from build123d import *

# Parameters (mm, degrees)
ESQUISSE1_R             = 2.1
BOSS_EXTRU_1_DEPTH      = 3
BOSS_EXTRU_2_START      = -50
ESQUISSE4_R             = 5
BOSS_EXTRU_2_DEPTH      = 10
ENL_V_MAT_EXTRU_1_DEPTH = 10


with BuildPart() as part:
    # Esquisse1 → Boss.-Extru.1 (new body)
    with BuildSketch(Plane.XY):
        with BuildLine():
            Line((-35, -45), (35, -45))
            ThreePointArc((35, -45), (42.071067812, -42.071067812), (45, -35))
            Line((45, -35), (45, 35))
            ThreePointArc((45, 35), (42.071067812, 42.071067812), (35, 45))
            Line((35, 45), (-35, 45))
            ThreePointArc((-35, 45), (-42.071067812, 42.071067812), (-45, 35))
            Line((-45, 35), (-45, -35))
            ThreePointArc((-45, -35), (-42.071067812, -42.071067812), (-35, -45))
        make_face()
        with Locations((-37.5, 37.5)):
            Circle(ESQUISSE1_R, mode=Mode.SUBTRACT)
        with Locations((37.5, 37.5)):
            Circle(ESQUISSE1_R, mode=Mode.SUBTRACT)
        with Locations((37.5, -37.5)):
            Circle(ESQUISSE1_R, mode=Mode.SUBTRACT)
        with Locations((-37.5, -37.5)):
            Circle(ESQUISSE1_R, mode=Mode.SUBTRACT)
    extrude(amount=BOSS_EXTRU_1_DEPTH)

    # Esquisse4 → Boss.-Extru.2 (add)
    with BuildSketch(Plane(origin=(0, 45, 123.316242038), x_dir=(1, 0, 0), z_dir=(0, 1, 0)).offset(BOSS_EXTRU_2_START)):
        with BuildLine():
            Line((10, 120.316242038), (10, 110.316242038))
            ThreePointArc((10, 110.316242038), (0, 100.316242038), (-10, 110.316242038))
            Line((-10, 110.316242038), (-10, 120.316242038))
            Line((-10, 120.316242038), (10, 120.316242038))
        make_face()
        with Locations((0, 110.316242038)):
            Circle(ESQUISSE4_R, mode=Mode.SUBTRACT)
    extrude(amount=BOSS_EXTRU_2_DEPTH)

    # Esquisse5 → Enlèv. mat.-Extru.1 (cut)
    with BuildSketch(Plane.XY.offset(3)):
        with BuildLine():
            Line((-23.186291501, 37.5), (23.186291501, 37.5))
            ThreePointArc((23.186291501, 37.5), (25.957930099, 35.648050297), (25.307611845, 32.378679656))
            Line((25.307611845, 32.378679656), (3.807611845, 10.878679656))
            ThreePointArc((3.807611845, 10.878679656), (2.834341798, 10.228361402), (1.686291501, 10))
            Line((1.686291501, 10), (-1.686291501, 10))
            ThreePointArc((-1.686291501, 10), (-2.834341798, 10.228361402), (-3.807611845, 10.878679656))
            Line((-3.807611845, 10.878679656), (-25.307611845, 32.378679656))
            ThreePointArc((-25.307611845, 32.378679656), (-25.957930099, 35.648050297), (-23.186291501, 37.5))
        make_face()
        with BuildLine():
            Line((-32.378679656, -25.307611845), (-10.878679656, -3.807611845))
            ThreePointArc((-10.878679656, -3.807611845), (-10.228361402, -2.834341798), (-10, -1.686291501))
            Line((-10, -1.686291501), (-10, 1.686291501))
            ThreePointArc((-10, 1.686291501), (-10.228361402, 2.834341798), (-10.878679656, 3.807611845))
            Line((-10.878679656, 3.807611845), (-32.378679656, 25.307611845))
            ThreePointArc((-32.378679656, 25.307611845), (-35.648050297, 25.957930099), (-37.5, 23.186291501))
            Line((-37.5, 23.186291501), (-37.5, -23.186291501))
            ThreePointArc((-37.5, -23.186291501), (-35.648050297, -25.957930099), (-32.378679656, -25.307611845))
        make_face()
        with BuildLine():
            Line((32.378679656, 25.307611845), (10.878679656, 3.807611845))
            ThreePointArc((10.878679656, 3.807611845), (10.228361402, 2.834341798), (10, 1.686291501))
            Line((10, 1.686291501), (10, -1.686291501))
            ThreePointArc((10, -1.686291501), (10.228361402, -2.834341798), (10.878679656, -3.807611845))
            Line((10.878679656, -3.807611845), (32.378679656, -25.307611845))
            ThreePointArc((32.378679656, -25.307611845), (35.648050297, -25.957930099), (37.5, -23.186291501))
            Line((37.5, -23.186291501), (37.5, 23.186291501))
            ThreePointArc((37.5, 23.186291501), (35.648050297, 25.957930099), (32.378679656, 25.307611845))
        make_face()
        with BuildLine():
            Line((23.186291501, -37.5), (-23.186291501, -37.5))
            ThreePointArc((-23.186291501, -37.5), (-25.957930099, -35.648050297), (-25.307611845, -32.378679656))
            Line((-25.307611845, -32.378679656), (-3.807611845, -10.878679656))
            ThreePointArc((-3.807611845, -10.878679656), (-2.834341798, -10.228361402), (-1.686291501, -10))
            Line((-1.686291501, -10), (1.686291501, -10))
            ThreePointArc((1.686291501, -10), (2.834341798, -10.228361402), (3.807611845, -10.878679656))
            Line((3.807611845, -10.878679656), (25.307611845, -32.378679656))
            ThreePointArc((25.307611845, -32.378679656), (25.957930099, -35.648050297), (23.186291501, -37.5))
        make_face()
    extrude(amount=-ENL_V_MAT_EXTRU_1_DEPTH, mode=Mode.SUBTRACT)


solid = part.part
Part model, mm, in its own coordinate system. A direction names the side the tool comes from. Give positions to 0.01 mm unless a question says otherwise; leave off trailing zeros. Loops run counter-clockwise (first coordinate to the right, second up) from the corner with the lowest first, then second, coordinate; pieces in that order, holes last. Notation, with made-up numbers: M 11,86.5 L 54,86.5 A24 cw 54,124.5 Z; hole C -20.5,59 d4. An arc over 180 degrees is marked long. Put each result on its own line as item: value. Start each with the question number.
1) Saw through at A-A (x = 0). List the corners of the cut face in (y, z), then the cut area to 3 significant figures.
2) Saw through at B-B (y = -13.5). List the corners of the cut face in (x, z).
3) Pull direction Y, two halves, no side cores. Call faces 1 (the cylindrical face through (41.99, -42.15, 1.48)), 2 (the cylindrical face through (-2.85, -10.235, 1.521)), 3 (the cylindrical face through (-35.602, 25.976, 1.521)), 4 (the cylindrical face through (42.15, 41.99, 1.48)): +Y half, -Y half, draft (parallel to the pull), parting line (faces both ways), or undercut.
4) 3-axis set-ups, long thin cutter, end or side, ignore diameter. For faces 5 (the flat face through (37.5, 0, 2)), 6 (the flat face through (0, -45, 1)), 7 (the flat face through (2, -5, 8)): which of +Z, -Z, +X, -X, +Y, -Y reach the whole face in a straight line?
5) Saw through at C-C (z = 14.75). List the corners of the cut face in (x, y), then the cut area to 3 significant figures.
6) Flat gauge pins, fed straight in: pin 1 (2 mm diameter, centred on x = -7.5, z = 7.5, fed in from -Y); pin 2 (6 mm diameter, centred on x = -4, z = 16, fed in from +Y); pin 3 (8 mm diameter, centred on y = -2.5, z = 8.5, fed in from -X). Where does each tip first touch, or does it go through?
7) Probe probe 1 along Z at (x, y) = (0, -2); probe 2 along X at (y, z) = (-8.5, 2.25); probe 3 along Z at (x, y) = (19, 25). List the from-to ranges inside material, lowest first.
8) Saw through at D-D (y = 33.5). List the corners of the cut face in (x, z), then the cut area to 3 significant figures.
Numbers:
1. outline: M -45,0 L -37.5,0 L -37.5,3 L -45,3 Z; M -10,0 L 10,0 L 10,3 L 5,3 L 5,8 L -5,8 L -5,3 L -10,3 Z; M -5,18 L 5,18 L 5,23 L -5,23 Z; M 37.5,0 L 45,0 L 45,3 L 37.5,3 Z
1. area: 205 mm^2
2. outline: M -45,0 L -37.5,0 L -37.5,3 L -45,3 Z; M -20.57,0 L -6.43,0 L -6.43,3 L -20.57,3 Z; M 6.43,0 L 20.57,0 L 20.57,3 L 6.43,3 Z; M 37.5,0 L 45,0 L 45,3 L 37.5,3 Z
3. face 1: -Y half
3. face 2: undercut
3. face 3: undercut
3. face 4: +Y half
4. face 5: +Z, -Z
4. face 6: +Z, -Z, +X, -X, -Y
4. face 7: +Z, +X, -X, -Y
5. outline: M -9.85,-5 L -4.68,-5 L -4.68,5 L -9.85,5 Z; M 4.68,-5 L 9.85,-5 L 9.85,5 L 4.68,5 Z
5. area: 103 mm^2
6. pin 1: y = -5
6. pin 2: y = 5
6. pin 3: x = -10
7. probe 1: 0 to 8, 18 to 23
7. probe 2: -45 to -37.5, -15.57 to 15.57, 37.5 to 45
7. probe 3: 0 to 3
8. outline: M -45,0 L -26.01,0 L -26.01,3 L -45,3 Z; M 26.01,0 L 45,0 L 45,3 L 26.01,3 Z
8. area: 114 mm^2
